Work out the finished part from the listing and answer in its coordinate system (mm). Round coordinates to 2 decimals unless told otherwise and drop trailing zeros. Loops run counter-clockwise (first coordinate to the right, second up) from the corner with the lowest first, then second, coordinate; pieces in that order, holes last. Notation, with made-up numbers: (-13.5, 43.25) - (45.5, 43.25) arc R24 cw to (45.5, 54.25) - close; hole circle Ø9 at (35.5, -36.75). An arc over 180 degrees is marked (long way). Return JSON: item names as keys, results as strings.
Autodesk Inventor part; units mm, degrees
ref_plane "YZ Plane" through (0, 0, 0) normal (1, 0, 0) x (0, 1, 0)
ref_plane "XZ Plane" through (0, 0, 0) normal (0, 1, 0) x (-1, 0, 0)
ref_plane "XY Plane" through (0, 0, 0) normal (0, 0, 1) x (1, 0, 0)
sketch "Sketch1" plane through (0, 0, 0) normal (0, 0, 1) x (1, 0, 0)
  circle A0 centre (0, 0) radius 13
  circle A1 centre (-6, 6) radius 1
  circle A2 centre (0, 6) radius 1
  circle A3 centre (6, 6) radius 1
  circle A4 centre (6, -6) radius 1
  circle A5 centre (0, -6) radius 1
  circle A6 centre (-6, -6) radius 1
  dimension "d0" = 26
  dimension "d2" = 2
  dimension "d3" = 12
  dimension "d4" = 6
  dimension "d5" = 12
  dimension "d6" = 6
  dimension "d7" = 6
  dimension "d8" = 2
extrude "Extrusion1" add sketch "Sketch1" along normal blind 1
sketch "Sketch2" plane through (0, 0, 1) normal (0, 0, -1) x (-1, 0, 0)
  circle A0 centre (4, 0) radius 5
  circle A1 centre (0, 6) radius 1
  point P0 (0, 0)
  dimension "d11" = 10
  dimension "d12" = 4
extrude "Extrusion2" cut sketch "Sketch2" along normal blind 18 contours A0
properties part number "12"
1) Section A-A (y = 0) is taken. Give the vertices of the cut face in (x, z).
Verdict:
{"outline": "(-13, 0) - (-9, 0) - (-9, 1) - (-13, 1) - close; (1, 0) - (13, 0) - (13, 1) - (1, 1) - close"}
2) Section D-D (y = 6) is taken. Give the vertices of the cut face in (x, z), and give its area (3 significant figures).
Verdict:
{"outline": "(-11.53, 0) - (-7, 0) - (-7, 1) - (-11.53, 1) - close; (-5, 0) - (-1, 0) - (-1, 1) - (-5, 1) - close; (1, 0) - (5, 0) - (5, 1) - (1, 1) - close; (7, 0) - (11.53, 0) - (11.53, 1) - (7, 1) - close", "area": "17.1 mm2"}
3) Determine the mould class of faces 1 (the flat face through (3, 0, 0)), 2 (the cylindrical face through (-10.316, 7.91, 0.493)), 3 (the cylindrical face through (-0.13, 5.01, 0.49)) for opening direction Y: pulls with the +Y half, pulls with the -Y half, needs draft (parallel to the pull), parting line crosses it, or undercut.
Verdict:
{"face 1": "needs draft", "face 2": "parting line crosses it", "face 3": "undercut"}
4) Section B-B (x = -3.25) is taken. Give the vertices of the cut face in (y, z), and give its area (3 significant figures).
Verdict:
{"outline": "(-12.59, 0) - (-4.94, 0) - (-4.94, 1) - (-12.59, 1) - close; (4.94, 0) - (12.59, 0) - (12.59, 1) - (4.94, 1) - close", "area": "15.3 mm2"}
5) Find the intervals of material crossed by L1, parallel to Y at x = 0, z = 0.3; L2, parallel to Y at x = 6, z = 0.4; L3, parallel to Y at x = -6, z = 0.85, in increasing order.
Verdict:
{"L1": "y = -13 to -7, -5 to -3, 3 to 5, 7 to 13", "L2": "y = -11.53 to -7, -5 to 5, 7 to 11.53", "L3": "y = -11.53 to -7, -5 to -4.58, 4.58 to 5, 7 to 11.53"}
6) Section C-C (z = 0.55) is taken. Give the vertices of the cut face in (x, y), and give its area (3 significant figures).
Verdict:
{"outline": "circle Ø26 at (0, 0); hole circle Ø10 at (-4, 0); hole circle Ø2 at (-6, -6); hole circle Ø2 at (-6, 6); hole circle Ø2 at (0, -6); hole circle Ø2 at (0, 6); hole circle Ø2 at (6, -6); hole circle Ø2 at (6, 6)", "area": "434 mm2"}
7) A flat-ended cylindrical pin translates along its axis: pin 1 (3 mm diameter, centred on x = -6, y = 6, fed in from +Z). Find the tip coordinate at first contact, or state that the pin passes through.
Verdict:
{"pin 1": "stops at z = 1"}
